from build123d import *
from build123d.topology import SkipClean

# Parameters (mm, degrees)
SKETCH1_R           = 18.5
BOSS_EXTRUDE1_DEPTH = 3.5
SKETCH2_R           = 35
SKETCH2_R_2         = 20
SKETCH2_R_3         = 2.8
BOSS_EXTRUDE2_DEPTH = 6
SKETCH5_R           = 5
BOSS_EXTRUDE4_DEPTH = 3
CUT_EXTRUDE1_START  = -10
SKETCH3_R           = 18.5
CUT_EXTRUDE1_DEPTH  = 10
SKETCH12_R          = 72.135852014
CUT_EXTRUDE2_DEPTH  = 22
FILLET1_R           = 10
SKETCH15_R          = 20
SKETCH15_R_2        = 6
CUT_EXTRUDE4_DEPTH  = 2
SKETCH4_R           = 3.2
CUT_EXTRUDE5_DEPTH  = 10


with BuildPart() as part:
    # Sketch1 → Boss-Extrude1 (new body)
    with BuildSketch(Plane(origin=(0, 0, 0), x_dir=(1, 0, 0), z_dir=(0, 1, 0))):
        with Locations(Location((0, 0, 0), (0, 0, 270))):
            Circle(SKETCH1_R)
    extrude(amount=BOSS_EXTRUDE1_DEPTH)

    # Sketch3 → Cut-Extrude1 (cut)
    with BuildSketch(Plane(origin=(0, 3.5, 0), x_dir=(1, 0, 0), z_dir=(0, 1, 0)).offset(CUT_EXTRUDE1_START)):
        Circle(SKETCH3_R)
    extrude(amount=CUT_EXTRUDE1_DEPTH, mode=Mode.SUBTRACT)


with BuildPart() as body_2:
    # Sketch2 → Boss-Extrude2 (new body)
    with BuildSketch(Plane(origin=(0, 0, 0), x_dir=(1, 0, 0), z_dir=(0, 1, 0))):
        with Locations(Location((0, 0, 0), (0, 0, 270))):
            Circle(SKETCH2_R)
        with Locations(Location((0, 0, 0), (0, 0, 270))):
            Circle(SKETCH2_R_2, mode=Mode.SUBTRACT)
        with Locations(Location((0, 29, 0), (0, 0, 270))):
            Circle(SKETCH2_R_3, mode=Mode.SUBTRACT)
        with Locations(Location((25.11473671, -14.5, 0), (0, 0, 270))):
            Circle(SKETCH2_R_3, mode=Mode.SUBTRACT)
        with Locations(Location((-25.11473671, -14.5, 0), (0, 0, 270))):
            Circle(SKETCH2_R_3, mode=Mode.SUBTRACT)
    extrude(amount=BOSS_EXTRUDE2_DEPTH)

    # Sketch5 → Boss-Extrude4 (add)
    with BuildSketch(Plane(origin=(0, 6, 0), x_dir=(1, 0, 0), z_dir=(0, 1, 0))):
        with Locations((-30.453629482, -17.250404383)):
            Circle(SKETCH5_R)
        with Locations((0.28752632, 34.99881896)):
            Circle(SKETCH5_R)
        with Locations((30.166103162, -17.748414577)):
            Circle(SKETCH5_R)
    extrude(amount=-BOSS_EXTRUDE4_DEPTH)

    # Sketch12 → Cut-Extrude2 (cut)
    with BuildSketch(Plane(origin=(0, 6, 0), x_dir=(1, 0, 0), z_dir=(0, 1, 0))):
        Circle(SKETCH12_R)
        Polygon((0, 50), (-43.301270189, -25), (43.301270189, -25), align=None, mode=Mode.SUBTRACT)
    extrude(amount=-CUT_EXTRUDE2_DEPTH, mode=Mode.SUBTRACT)

    # Fillet1
    # the kernel refuses this fillet: 10 mm, written as the material it takes off along each edge
    with BuildSketch(Plane(origin=(-24.494897428, 19.2960859, 25), x_dir=(-0.6590478202651217, 0, -0.7521010374968192), z_dir=(0, -1, 0))) as fillet1_piece_1_section:
        with BuildLine():
            CenterArc((4.558658023, 9.971095222), FILLET1_R, 221.227294524, 53.130102354)
            Line((-2.962352352, 3.380617019), (0, 0))
            ThreePointArc((0, 0), (2.65921718, -0.101166725), (5.31843436, 0))
        make_face()
    fillet1_piece_1 = extrude(amount=32.5921718, mode=Mode.PRIVATE)
    fillet1_piece_1 = fillet1_piece_1 - Plane(origin=(-30.453629482, 4.5, 17.250404383), x_dir=(1, 0, 0), z_dir=(0, 1, 0)) * Cylinder(5, 87, mode=Mode.PRIVATE)
    add(fillet1_piece_1, mode=Mode.SUBTRACT)
    with BuildSketch(Plane(origin=(-24.494897428, 19.2960859, 25), x_dir=(-0.6590478202651217, 0, -0.7521010374968192), z_dir=(0, -1, 0))) as fillet1_piece_2_section:
        with BuildLine():
            CenterArc((4.558658023, 9.971095222), FILLET1_R, 221.227294524, 53.130102354)
            Line((-2.962352352, 3.380617019), (0, 0))
            ThreePointArc((0, 0), (2.65921718, -0.101166725), (5.31843436, 0))
        make_face()
    fillet1_piece_2 = extrude(amount=32.5921718, mode=Mode.PRIVATE)
    fillet1_piece_2 = split(fillet1_piece_2, bisect_by=Plane(origin=(-27.761621835, 3, 21.309124186), z_dir=(0, -1, 0)), keep=Keep.TOP, mode=Mode.PRIVATE)
    add(fillet1_piece_2, mode=Mode.SUBTRACT)
    with BuildSketch(Plane(origin=(24.494897428, 19.2960859, 25), x_dir=(-1, 0, 0), z_dir=(0, -1, 0))) as fillet1_piece_3_section:
        with BuildLine():
            CenterArc((4.494897428, 10), FILLET1_R, 216.869897646, 53.130102354)
            ThreePointArc((-3.505102572, 4), (-1.828638885, 1.933326291), (0, 0))
            Line((0, 0), (4.494897428, 0))
        make_face()
    fillet1_piece_3 = extrude(amount=32.5921718, mode=Mode.PRIVATE)
    fillet1_piece_3 = fillet1_piece_3 - Plane(origin=(30.166103162, 4.5, 17.748414577), x_dir=(1, 0, 0), z_dir=(0, 1, 0)) * Cylinder(5, 84, mode=Mode.PRIVATE)
    add(fillet1_piece_3, mode=Mode.SUBTRACT)
    with BuildSketch(Plane(origin=(24.494897428, 19.2960859, 25), x_dir=(-1, 0, 0), z_dir=(0, -1, 0))) as fillet1_piece_4_section:
        with BuildLine():
            CenterArc((4.494897428, 10), FILLET1_R, 216.869897646, 53.130102354)
            ThreePointArc((-3.505102572, 4), (-1.828638885, 1.933326291), (0, 0))
            Line((0, 0), (4.494897428, 0))
        make_face()
    fillet1_piece_4 = extrude(amount=32.5921718, mode=Mode.PRIVATE)
    fillet1_piece_4 = split(fillet1_piece_4, bisect_by=Plane(origin=(27.488157838, 3, 21.643747381), z_dir=(0, -1, 0)), keep=Keep.TOP, mode=Mode.PRIVATE)
    add(fillet1_piece_4, mode=Mode.SUBTRACT)
    with BuildSketch(Plane(origin=(-9.403186381, 19.2960859, -33.713203436), x_dir=(-0.5000000000000003, 0, 0.8660254037844386), z_dir=(0, -1, 0))) as fillet1_piece_5_section:
        with BuildLine():
            CenterArc((4.494897428, -10), FILLET1_R, 90, 53.130102354)
            ThreePointArc((-3.505102572, -4), (-1.828638885, -1.933326291), (0, 0))
            Line((0, 0), (4.494897428, 0))
        make_face()
    fillet1_piece_5 = extrude(amount=32.5921718, mode=Mode.PRIVATE)
    fillet1_piece_5 = fillet1_piece_5 - Plane(origin=(0.28752632, 4.5, -34.99881896), x_dir=(1, 0, 0), z_dir=(0, 1, 0)) * Cylinder(5, 84, mode=Mode.PRIVATE)
    add(fillet1_piece_5, mode=Mode.SUBTRACT)
    with BuildSketch(Plane(origin=(-9.403186381, 19.2960859, -33.713203436), x_dir=(-0.5000000000000003, 0, 0.8660254037844386), z_dir=(0, -1, 0))) as fillet1_piece_6_section:
        with BuildLine():
            CenterArc((4.494897428, -10), FILLET1_R, 90, 53.130102354)
            ThreePointArc((-3.505102572, -4), (-1.828638885, -1.933326291), (0, 0))
            Line((0, 0), (4.494897428, 0))
        make_face()
    fillet1_piece_6 = extrude(amount=32.5921718, mode=Mode.PRIVATE)
    fillet1_piece_6 = split(fillet1_piece_6, bisect_by=Plane(origin=(-4.57343196, 3, -34.696831852), z_dir=(0, -1, 0)), keep=Keep.TOP, mode=Mode.PRIVATE)
    add(fillet1_piece_6, mode=Mode.SUBTRACT)
    with BuildSketch(Plane(origin=(-33.898083809, 19.2960859, 8.713203436), x_dir=(0.32181469455231854, 0, 0.9468026734067654), z_dir=(0, -1, 0))) as fillet1_piece_7_section:
        with BuildLine():
            CenterArc((4.558658023, -9.971095222), FILLET1_R, 85.642603122, 53.130102354)
            Line((-2.962352352, -3.380617019), (0, 0))
            ThreePointArc((0, 0), (2.65921718, 0.101166725), (5.31843436, 0))
        make_face()
    fillet1_piece_7 = extrude(amount=32.5921718, mode=Mode.PRIVATE)
    fillet1_piece_7 = fillet1_piece_7 - Plane(origin=(-30.453629482, 4.5, 17.250404383), x_dir=(1, 0, 0), z_dir=(0, 1, 0)) * Cylinder(5, 87, mode=Mode.PRIVATE)
    add(fillet1_piece_7, mode=Mode.SUBTRACT)
    with BuildSketch(Plane(origin=(-33.898083809, 19.2960859, 8.713203436), x_dir=(0.32181469455231854, 0, 0.9468026734067654), z_dir=(0, -1, 0))) as fillet1_piece_8_section:
        with BuildLine():
            CenterArc((4.558658023, -9.971095222), FILLET1_R, 85.642603122, 53.130102354)
            Line((-2.962352352, -3.380617019), (0, 0))
            ThreePointArc((0, 0), (2.65921718, 0.101166725), (5.31843436, 0))
        make_face()
    fillet1_piece_8 = extrude(amount=32.5921718, mode=Mode.PRIVATE)
    fillet1_piece_8 = split(fillet1_piece_8, bisect_by=Plane(origin=(-32.488113984, 3, 12.9835693), z_dir=(0, -1, 0)), keep=Keep.TOP, mode=Mode.PRIVATE)
    add(fillet1_piece_8, mode=Mode.SUBTRACT)
    with BuildSketch(Plane(origin=(33.898083809, 19.2960859, 8.713203436), x_dir=(-0.3218146945523175, 0, 0.9468026734067657), z_dir=(0, -1, 0))) as fillet1_piece_9_section:
        with BuildLine():
            CenterArc((4.558658023, 9.971095222), FILLET1_R, 221.227294524, 53.130102354)
            Line((-2.962352352, 3.380617019), (0, 0))
            ThreePointArc((0, 0), (2.65921718, -0.101166725), (5.31843436, 0))
        make_face()
    fillet1_piece_9 = extrude(amount=32.5921718, mode=Mode.PRIVATE)
    fillet1_piece_9 = fillet1_piece_9 - Plane(origin=(30.166103162, 4.5, 17.748414577), x_dir=(1, 0, 0), z_dir=(0, 1, 0)) * Cylinder(5, 87, mode=Mode.PRIVATE)
    add(fillet1_piece_9, mode=Mode.SUBTRACT)
    with BuildSketch(Plane(origin=(33.898083809, 19.2960859, 8.713203436), x_dir=(-0.3218146945523175, 0, 0.9468026734067657), z_dir=(0, -1, 0))) as fillet1_piece_10_section:
        with BuildLine():
            CenterArc((4.558658023, 9.971095222), FILLET1_R, 221.227294524, 53.130102354)
            Line((-2.962352352, 3.380617019), (0, 0))
            ThreePointArc((0, 0), (2.65921718, -0.101166725), (5.31843436, 0))
        make_face()
    fillet1_piece_10 = extrude(amount=32.5921718, mode=Mode.PRIVATE)
    fillet1_piece_10 = split(fillet1_piece_10, bisect_by=Plane(origin=(32.335053795, 3, 13.387707666), z_dir=(0, -1, 0)), keep=Keep.TOP, mode=Mode.PRIVATE)
    add(fillet1_piece_10, mode=Mode.SUBTRACT)
    with BuildSketch(Plane(origin=(9.403186381, 19.2960859, -33.713203436), x_dir=(-0.9808625148174394, 0, -0.19470163590994477), z_dir=(0, -1, 0))) as fillet1_piece_11_section:
        with BuildLine():
            CenterArc((4.558658023, -9.971095222), FILLET1_R, 85.642603122, 53.130102354)
            Line((-2.962352352, -3.380617019), (0, 0))
            ThreePointArc((0, 0), (2.65921718, 0.101166725), (5.31843436, 0))
        make_face()
    fillet1_piece_11 = extrude(amount=32.5921718, mode=Mode.PRIVATE)
    fillet1_piece_11 = fillet1_piece_11 - Plane(origin=(0.28752632, 4.5, -34.99881896), x_dir=(1, 0, 0), z_dir=(0, 1, 0)) * Cylinder(5, 87, mode=Mode.PRIVATE)
    add(fillet1_piece_11, mode=Mode.SUBTRACT)
    with BuildSketch(Plane(origin=(9.403186381, 19.2960859, -33.713203436), x_dir=(-0.9808625148174394, 0, -0.19470163590994477), z_dir=(0, -1, 0))) as fillet1_piece_12_section:
        with BuildLine():
            CenterArc((4.558658023, -9.971095222), FILLET1_R, 85.642603122, 53.130102354)
            Line((-2.962352352, -3.380617019), (0, 0))
            ThreePointArc((0, 0), (2.65921718, 0.101166725), (5.31843436, 0))
        make_face()
    fillet1_piece_12 = extrude(amount=32.5921718, mode=Mode.PRIVATE)
    fillet1_piece_12 = split(fillet1_piece_12, bisect_by=Plane(origin=(4.999956146, 3, -34.627316681), z_dir=(0, -1, 0)), keep=Keep.TOP, mode=Mode.PRIVATE)
    add(fillet1_piece_12, mode=Mode.SUBTRACT)

    # Sketch15 → Cut-Extrude4 (cut)
    with SkipClean():  # the faces are left unmerged after this step: merging them gives an invalid solid
        with BuildSketch(Plane(origin=(0, 6, 0), x_dir=(1, 0, 0), z_dir=(0, 1, 0))):
            with Locations(Location((0, 0, 0), (0, 0, 107.923924211))):
                Circle(SKETCH15_R)
            with Locations((-9.237551188, -16.028650849)):
                Circle(SKETCH15_R_2)
            with Locations((18.499994418, 0.014371427)):
                Circle(SKETCH15_R_2)
            with BuildLine():
                Line((-12.266478871, 21.208099776), (-13.42538307, 14.824273656))
                ThreePointArc((-13.42538307, 14.824273656), (-10.01345214, 17.312734511), (-6.155078704, 19.029319645))
                Line((-6.155078704, 19.029319645), (-12.266478871, 21.208099776))
            make_face()
        extrude(amount=-CUT_EXTRUDE4_DEPTH, mode=Mode.SUBTRACT)

    # Sketch4 → Cut-Extrude5 (cut)
    with SkipClean():  # the faces are left unmerged after this step: merging them gives an invalid solid
        with BuildSketch(Plane.XZ):
            with Locations(Location((-25.11473671, 14.5, 0), (0, 0, 270))):
                Circle(SKETCH4_R)
            with Locations(Location((25.11473671, 14.5, 0), (0, 0, 270))):
                Circle(SKETCH4_R)
            with Locations(Location((0, -29, 0), (0, 0, 270))):
                Circle(SKETCH4_R)
        extrude(amount=-CUT_EXTRUDE5_DEPTH, mode=Mode.SUBTRACT)


solid = body_2.part
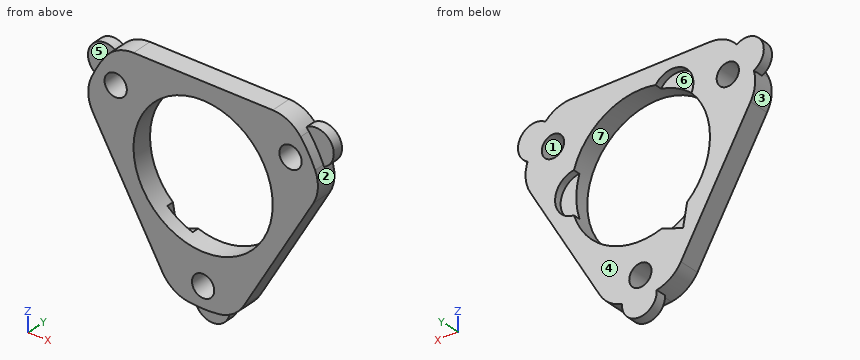
Geometry: final body of the model. Coordinates: model frame, mm. Face numbers are marked on the shaded views. A direction names the side the tool comes from. Coordinates: 2 decimals unless noted, no trailing zeros. Order: outer loops, then holes, each group sorted by start corner. A loop starts at its lowest first (then second) coordinate and runs counter-clockwise, first axis right, second up. Notation, with made-up numbers: M -14.75,86.25 L 42.25,86.25 A25 ccw 42.25,100.25 Z; hole C -34,-29 d10. An arc over 180 degrees is marked long. One line per question, with ' | ' between items. Start each with the question number.
Item 1: Cut plane B-B, the plane x = 6.5. Return the cut outline in (y, z).
Item 2: Ray query, probe 1 along X at (y, z) = (4.2, 14.5); probe 2 along Z at (x, y) = (-16.5, 0.75); probe 3 along X at (y, z) = (1.25, 5). Return the intervals inside material, ascending. Write a range as [from, to].
Item 3: Cut plane A-A, the plane z = -29. Return the cut outline in (x, y).
Item 4: Pin query (flat end, axial travel): pin 1 Ø4.5 at (x, z) = (21, -2.5) entering from +Y; pin 2 Ø1 at (x, y) = (-16, 2) entering from -Z; pin 3 Ø4 at (x, z) = (25.11, 14.5) entering from -Y; pin 4 Ø4 at (x, z) = (32.5, 18.5) entering from -Y. Return the tip coordinate at first contact, or that it passes through.
Item 5: Draft query along X for the marked faces 1, 2, 3 and 4. Return one class per face: released by +X, released by -X, zero draft, split by the parting line, or undercut.
Item 6: Cut plane D-D, the plane z = -1.5. Return the cut outline in (x, y).
Item 7: Set-up query: the marked faces 5, 6 and 7. Return all of +Z, -Z, +X, -X, +Y, -Y with unobstructed straight access to the full face (end or side cutting, diameter ignored); none if empty.
Item 8: Cut plane C-C, the plane y = 1.75. Return the cut outline in (x, z).
A:
1) outline: M 0,-34.18 L 6,-34.18 L 6,-18.91 L 0,-18.91 Z; M 0,18.91 L 6,18.91 L 6,25 L 0,25 Z
2) probe 1: x = [-34.63, -28.31], [-21.91, -15.04], [13.77, 21.91], [28.31, 33.97] | probe 2: z = [-21.42, -11.3], [11.3, 25] | probe 3: x = [-31.75, -19.36], [19.36, 31.75]
3) outline: M -12.12,0 L -3.2,0 L -3.2,6 L -12.12,6 Z; M 3.2,0 L 12.12,0 L 12.12,6 L 3.2,6 Z
4) pin 1: stops at y = 4 | pin 2: stops at z = -23.15 | pin 3: passes through | pin 4: stops at y = 3
5) face 1: undercut | face 2: released by +X | face 3: released by -X | face 4: zero draft
6) outline: M -28,0 L -19.94,0 L -19.94,6 L -28,6 Z; M 19.94,0 L 28,0 L 28,6 L 24.31,6 L 24.31,4 L 19.94,4 Z
7) face 5: +Z, -X, -Y | face 6: +Y | face 7: +Y, -Y
8) outline: M -32.19,13.75 A10 ccw -31.65,4.82 L -11.65,-29.82 A10 ccw -4.19,-34.75 A35 ccw 4.19,-34.75 A10 ccw 11.65,-29.82 L 31.65,4.82 A10 ccw 32.19,13.75 A35 ccw 28,21 A10 ccw 20,25 L -20,25 A10 ccw -28,21 A35 ccw Z; hole C -25.11,14.5 d6.4; hole C 0,0 d40; hole C 0,-29 d6.4; hole C 25.11,14.5 d6.4
